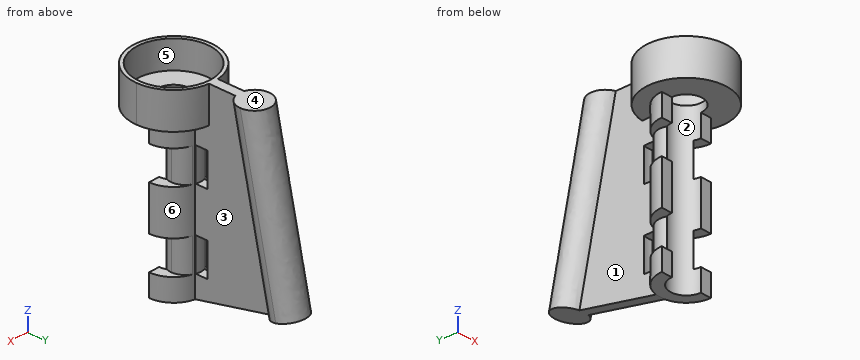
from build123d import *

# Parameters (mm, degrees)
F1_DEPTH    = 44.45
F9_DEPTH    = 9.525
F10_DEPTH   = 9.525
F12_DEPTH   = 2.38125
F13_R       = 11.7475
F13_R_2     = 10.7315
F14_DEPTH   = 7.9375
F15_DEPTH   = 10.31875
F15_FACE1_W = 2.794
F15_FACE1_H = 54.76875
F22_DEPTH   = 12.7


with BuildPart() as f1:
    # F0 (on Top) → F1 (new body)
    with BuildSketch(Plane.XY):
        with BuildLine():
            ThreePointArc((-4.572, 0), (0, 4.572), (4.572, 0))
            Line((4.572, 0), (7.747, 0))
            ThreePointArc((7.747, 0), (5.951410253, 4.9595085442), (1.397, 7.62))
            ThreePointArc((1.397, 7.62), (0, 7.747), (-1.397, 7.62))
            ThreePointArc((-1.397, 7.62), (-5.951410253, 4.9595085442), (-7.747, 0))
            Line((-7.747, 0), (-4.572, 0))
        make_face()
        with BuildLine():
            ThreePointArc((-1.397, 7.62), (0, 7.747), (1.397, 7.62))
            Line((1.397, 7.62), (1.397, 19.3802))
            Line((1.397, 19.3802), (-1.397, 19.3802))
            Line((-1.397, 19.3802), (-1.397, 7.62))
        make_face()
    extrude(amount=F1_DEPTH)

    # F6 (on offset) → F9 (cut)
    with BuildSketch(Plane.XY.offset(28.575)):
        with BuildLine():
            ThreePointArc((4.1557772601, 1.7640375299), (0, -1.016), (-4.1557772601, 1.7640375299))
            Line((-4.1557772601, 1.7640375299), (-7.6070004234, 1.7640375299))
            ThreePointArc((-7.6070004234, 1.7640375299), (0, -4.318), (7.6070004234, 1.7640375299))
            Line((7.6070004234, 1.7640375299), (4.1557772601, 1.7640375299))
        make_face()
        with BuildLine():
            ThreePointArc((-4.1557772601, 1.7640375299), (-0.8747878771, 7.8904367738), (4.4961791045, 3.4801791045))
            ThreePointArc((4.4961791045, 3.4801791045), (4.4102576693, 2.6053912274), (4.1557772601, 1.7640375299))
            Line((4.1557772601, 1.7640375299), (7.6070004234, 1.7640375299))
            ThreePointArc((7.6070004234, 1.7640375299), (7.750237064, 2.6168003938), (7.7981791045, 3.4801791045))
            ThreePointArc((7.7981791045, 3.4801791045), (-0.8633787106, 11.2304161684), (-7.6070004234, 1.7640375299))
            Line((-7.6070004234, 1.7640375299), (-4.1557772601, 1.7640375299))
        make_face()
        with BuildLine():
            ThreePointArc((7.6070004234, 1.7640375299), (0, -4.318), (-7.6070004234, 1.7640375299))
            Line((-7.6070004234, 1.7640375299), (-8.4216929972, 1.7640375299))
            Line((-8.4216929972, 1.7640375299), (-8.4216929972, -6.3198274001))
            Line((-8.4216929972, -6.3198274001), (11.7628639564, -6.3198274001))
            Line((11.7628639564, -6.3198274001), (11.7628639564, 1.7640375299))
            Line((11.7628639564, 1.7640375299), (7.6070004234, 1.7640375299))
        make_face()
    extrude(amount=F9_DEPTH, mode=Mode.SUBTRACT)

    # F8 (on offset) → F10 (cut)
    with BuildSketch(Plane.XY.offset(15.875)):
        with BuildLine():
            ThreePointArc((4.179462045, 1.8225532258), (0, -1.016), (-4.179462045, 1.8225532258))
            Line((-4.179462045, 1.8225532258), (-7.6199654718, 1.8225532258))
            ThreePointArc((-7.6199654718, 1.8225532258), (0, -4.318), (7.6199654718, 1.8225532258))
            Line((7.6199654718, 1.8225532258), (4.179462045, 1.8225532258))
        make_face()
        with BuildLine():
            ThreePointArc((-4.179462045, 1.8225532258), (-0.8438058499, 7.8964692022), (4.4961791045, 3.4801791045))
            ThreePointArc((4.4961791045, 3.4801791045), (4.4162900977, 2.6363732546), (4.179462045, 1.8225532258))
            Line((4.179462045, 1.8225532258), (7.6199654718, 1.8225532258))
            ThreePointArc((7.6199654718, 1.8225532258), (7.7534976902, 2.6465899292), (7.7981791045, 3.4801791045))
            ThreePointArc((7.7981791045, 3.4801791045), (-0.8335891753, 11.2336767947), (-7.6199654718, 1.8225532258))
            Line((-7.6199654718, 1.8225532258), (-4.179462045, 1.8225532258))
        make_face()
        with BuildLine():
            ThreePointArc((7.6199654718, 1.8225532258), (0, -4.318), (-7.6199654718, 1.8225532258))
            Line((-7.6199654718, 1.8225532258), (-8.5849482566, 1.8225532258))
            Line((-8.5849482566, 1.8225532258), (-8.5849482566, -5.9901881032))
            Line((-8.5849482566, -5.9901881032), (8.4006469697, -5.9901881032))
            Line((8.4006469697, -5.9901881032), (8.4006469697, 1.8225532258))
            Line((8.4006469697, 1.8225532258), (7.6199654718, 1.8225532258))
        make_face()
    extrude(amount=-F10_DEPTH, mode=Mode.SUBTRACT)

    # F11 (on face) → F12 (join)
    with BuildSketch(Plane.XY.offset(44.45)):
        with BuildLine():
            ThreePointArc((-1.397, 11.6641393703), (-7.7971949684, -8.7867802337), (11.7475, 0))
            ThreePointArc((11.7475, 0), (8.7867802337, 7.7971949684), (1.397, 11.6641393703))
            Line((1.397, 11.6641393703), (1.397, 7.62))
            ThreePointArc((1.397, 7.62), (5.951410253, 4.9595085442), (7.747, 0))
            Line((7.747, 0), (4.572, 0))
            ThreePointArc((4.572, 0), (0, -4.572), (-4.572, 0))
            Line((-4.572, 0), (-7.747, 0))
            ThreePointArc((-7.747, 0), (-5.951410253, 4.9595085442), (-1.397, 7.62))
            Line((-1.397, 7.62), (-1.397, 11.6641393703))
        make_face()
        with BuildLine():
            Line((1.397, 7.62), (1.397, 11.6641393703))
            ThreePointArc((1.397, 11.6641393703), (0, 11.7475), (-1.397, 11.6641393703))
            Line((-1.397, 11.6641393703), (-1.397, 7.62))
            ThreePointArc((-1.397, 7.62), (-5.951410253, 4.9595085442), (-7.747, 0))
            Line((-7.747, 0), (-4.572, 0))
            ThreePointArc((-4.572, 0), (0, 4.572), (4.572, 0))
            Line((4.572, 0), (7.747, 0))
            ThreePointArc((7.747, 0), (5.951410253, 4.9595085442), (1.397, 7.62))
        make_face()
    extrude(amount=F12_DEPTH)

    # F13 (on face) → F14 (join)
    with BuildSketch(Plane.XY.offset(46.83125)):
        Circle(F13_R)
        Circle(F13_R_2, mode=Mode.SUBTRACT)
    extrude(amount=F14_DEPTH)

    # F15 (add, through all): a face of the model
    f15_faces = [f1.faces().sort_by_distance(p)[0] for p in [
        (0, 15.5499360639, 44.45),
    ]]
    extrude(f15_faces, amount=F15_DEPTH)

    # F18: sweep along a path in F17
    with BuildLine(Plane.YZ) as f18_path:
        Line((23.7335406713, 54.76875), (35.3749978582, 0))
    # F16 (on face) → F18 (sweep)
    with BuildSketch(Plane.XY.offset(54.76875)):
        with BuildLine():
            ThreePointArc((1.397, 19.3802), (3.6939320514, 21.0394638349), (4.572, 23.7335406713))
            ThreePointArc((4.572, 23.7335406713), (-2.6940768363, 27.4274727226), (-1.397, 19.3802))
            Line((-1.397, 19.3802), (1.397, 19.3802))
        make_face()
    sweep(path=f18_path.line)

    # F15_face1 (on face) → F19 (join, up to the next surface of F1)
    with BuildSketch(Plane(origin=(0, 19.3802, 27.384375), x_dir=(-1, 0, 0), z_dir=(0, 1, 0))):
        Rectangle(F15_FACE1_W, F15_FACE1_H)
    extrude(until=Until.NEXT)

    # F20: union 

    # F21 (on Right) → F22 (cut, symmetric)
    with BuildSketch(Plane.YZ):
        Polygon((39.6406120252, 6.8061911946), (7.62, 0), (8.2477421489, -2.2532611279), (41.5662580615, -2.2532611279), align=None)
    extrude(amount=F22_DEPTH, both=True, mode=Mode.SUBTRACT)


solid = f1.part
Model file for the job. Use its own axes, mm. Face numbers are marked on the shaded views. A direction names the side the tool comes from. Round coordinates to 2 decimals unless told otherwise and drop trailing zeros. Order: outer loops, then holes, each group sorted by start corner. A loop starts at its lowest first (then second) coordinate and runs counter-clockwise, first axis right, second up.
(1) Pull direction X, two halves, no side cores. Call the marked faces 1, 2 and 3: released by +X, released by -X, zero draft, split by the parting line, or undercut.
(2) 3-axis set-ups, long thin cutter, end or side, ignore diameter. For the marked faces 4, 5 and 6: which of +Z, -Z, +X, -X, +Y, -Y reach the whole face in a straight line?
(3) Pin check, flat tips, straight feed: pin 1 (3 mm diameter, centred on x = 5, y = 4.5, fed in from -Z); pin 2 (1 mm diameter, centred on x = -3, y = -6, fed in from +Z); pin 3 (12 mm diameter, centred on x = -0.5, z = 7, fed in from -Y); pin 4 (3 mm diameter, centred on x = 2.5, z = 38, fed in from -Y). Stop position of each tip, or through.
(4) Band-saw the part on B-B (y = -3). List the corners of the cut face in (x, z).
(5) Band-saw the part on C-C (x = -8.75). List the corners of the cut face in (y, z).
(6) Band-saw the part on D-D (y = 15.5). List the corners of the cut face in (x, z), then the cut area to 3 significant figures.
(7) Band-saw the part on A-A (x = 0). Give the number of separate pieces and of enclosed holes in the cut face, then the cut area to 3 significant figures.
(8) Drill centre lines: line 1 (Z direction, x = -7.5, y = 0.5) (3 decimals); line 2 (Z direction, x = -0.75, y = 9) (3 decimals); line 3 (Y direction, x = 0, z = 51). Where is each one in solid material? Low to high.
Verdict:
1. face 1: released by -X
1. face 2: undercut
1. face 3: released by +X
2. face 4: +Z, +X, -X, +Y, -Y
2. face 5: +Z
2. face 6: -Z, +X
3. pin 1: stops at z = 0
3. pin 2: stops at z = 46.83
3. pin 3: stops at y = 0
3. pin 4: stops at y = 2.21
4. outline: (-11.36, 44.45) - (-3.45, 44.45) - (-3.45, 46.83) - (-10.3, 46.83) - (-10.3, 54.77) - (-11.36, 54.77) - close; (3.45, 44.45) - (11.36, 44.45) - (11.36, 54.77) - (10.3, 54.77) - (10.3, 46.83) - (3.45, 46.83) - close
5. outline: (-7.84, 44.45) - (7.84, 44.45) - (7.84, 54.77) - (6.21, 54.77) - (6.21, 46.83) - (-6.21, 46.83) - (-6.21, 54.77) - (-7.84, 54.77) - close
6. outline: (-1.4, 1.67) - (1.4, 1.67) - (1.4, 54.77) - (-1.4, 54.77) - close
6. area: 148 mm2
7. separate pieces: 2
7. enclosed holes: 2
7. area: 1,430 mm2
8. line 1: z = 0 to 6.35, 15.875 to 28.575, 38.1 to 46.831
8. line 2: z = 0.293 to 6.35, 15.875 to 28.575, 38.1 to 46.831
8. line 3: y = -11.75 to -10.73, 10.73 to 29.11
